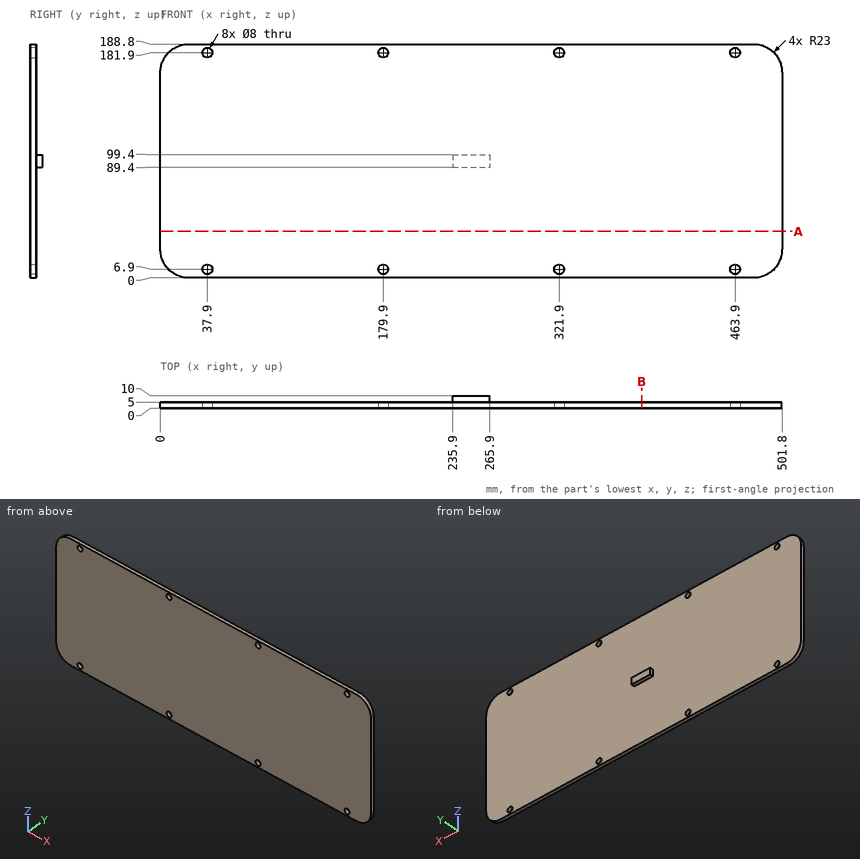
Study the drawing (mm; zero at the part's minimum x, y, z) and answer. Coordinates: 2 decimals unless noted, no trailing zeros. Loops run counter-clockwise (first coordinate to the right, second up) from the corner with the lowest first, then second, coordinate; pieces in that order, holes last. Notation, with made-up numbers: (-35, -5) -> (8, -5) arc R15 cw to (8, 24) -> close; hole circle Ø3 at (86, -20.75). An arc over 180 degrees is marked (long way). Answer in a Markdown table with one row per item. Add a question column.
1. The part is cut by section B-B, the plane x = 388.5. Write down the section's boundary in (y, z).
2. Consider line 1 (Z direction, x = 39, y = 1.75); line 2 (X direction, y = 4.05, z = 181.9); line 3 (Y direction, x = 278, z = 142). Determine where each line is inside the solid, lowest interval first. Write a range as [from, to].
3. The part is cut by section A-A, the plane z = 37.5. Write down the section's boundary in (x, y).
4. Flat-ended cylindrical pins translate along their axes: P1, Ø6, axis at x = 388.5, z = 136, coming from the +Y side; P2, Ø2, axis at x = 354.5, z = 161, coming from the -Y side; P3, Ø6.5, axis at x = 463.9, z = 181.9, coming from the -Y side; P4, Ø2.5, axis at x = 244.5, y = 7.5, coming from the -Z side. Find the tip coordinate at first contact, or state that the pin passes through.
Answer below:
| question | item | result |
|---|---|---|
| 1 | outline | (0, 0) -> (5, 0) -> (5, 188.8) -> (0, 188.8) -> close |
| 2 | line 1 | [0, 3.05], [10.75, 178.05], [185.75, 188.8] |
| 2 | line 2 | [6.57, 33.9], [41.9, 175.9], [183.9, 317.9], [325.9, 459.9], [467.9, 495.23] |
| 2 | line 3 | [0, 5] |
| 3 | outline | (0, 0) -> (501.8, 0) -> (501.8, 5) -> (0, 5) -> close |
| 4 | P1 | y = 5 |
| 4 | P2 | y = 0 |
| 4 | P3 | through |
| 4 | P4 | z = 89.4 |
